Source: three-view drawing plus pictorial views. Frame: mm from the lowest corner of the part. A direction names the side the tool comes from. Round coordinates to 2 decimals unless told otherwise and drop trailing zeros. Write each loop counter-clockwise with the first axis right and the second up, starting at its lowest first coordinate (ties: lowest second). Pieces come first, ordered by that corner, then holes. Notation, with made-up numbers: M 81,43 L 123,43 A20 cw 123,69 Z; hole C 49.25,89 d4. An arc over 180 degrees is marked long. Answer as CSV lines item,"result". Start each with the question number.
Q1. Section query D-D on x = 41. Output: boundary loops of the cut face in (y, z).
Q2. Mould query, pull axis X, two halves, no side actions, for the marked faces 1 and 2. Classes: pulls with the +X half, pulls with the -X half, needs draft (parallel to the pull), parting line crosses it, or undercut.
Q3. First-contact query: pin 1 (3.5 mm diameter, centred on x = 31, y = 3.5, fed in from -Z); pin 2 (1 mm diameter, centred on y = 5, z = 5.5, fed in from -X). Flat tips, straight axial feed; report the tip coordinate or a pass-through.
Q4. Section query A-A on y = 3.5. Output: boundary loops of the cut face in (x, z).
Q5. Reachability of the marked faces 3 and 4 from +Z, -Z, +X, -X, +Y, -Y: full face, straight path, thin tool, end or side. Return the list, or none.
Q6. Section query B-B on z = 9.5. Output: boundary loops of the cut face in (x, y), and give its area (3 significant figures).
Q7. Ray query, probe 1 along Y at (x, z) = (21, 6.5); probe 2 along X at (y, z) = (2.5, 5); probe 3 along X at (y, z) = (3, 6.5). Return the intervals inside material, ascending.
Q8. Section query C-C on x = 34. Output: boundary loops of the cut face in (y, z), and give its area (3 significant figures).
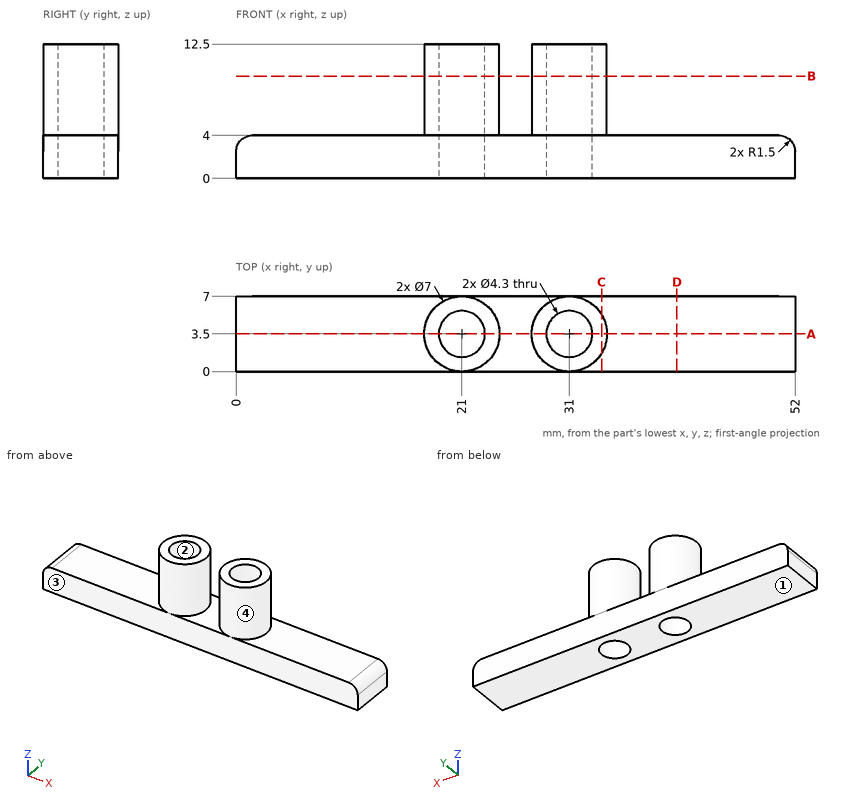
Entries:
1,outline,"M 0,0 L 7,0 L 7,4 L 0,4 Z"
2,face 1,"needs draft"
2,face 2,"undercut"
3,pin 1,"passes through"
3,pin 2,"stops at x = 17.65"
4,outline,"M 0,0 L 18.85,0 L 18.85,12.5 L 17.5,12.5 L 17.5,4 L 1.5,4 A1.5 ccw 0,2.5 Z; M 23.15,0 L 28.85,0 L 28.85,12.5 L 27.5,12.5 L 27.5,4 L 24.5,4 L 24.5,12.5 L 23.15,12.5 Z; M 33.15,0 L 52,0 L 52,2.5 A1.5 ccw 50.5,4 L 34.5,4 L 34.5,12.5 L 33.15,12.5 Z"
5,face 3,"+Z, -Z, +X, -X, -Y"
5,face 4,"+Z"
6,outline,"C 21,3.5 d7; C 31,3.5 d7; hole C 21,3.5 d4.3; hole C 31,3.5 d4.3"
6,area,"47.9 mm^2"
7,probe 1,"y = 0 to 1.35, 5.65 to 7"
7,probe 2,"x = 17.65 to 19.1, 22.9 to 24.35, 27.65 to 29.1, 32.9 to 34.35"
7,probe 3,"x = 17.54 to 18.91, 23.09 to 24.46, 27.54 to 28.91, 33.09 to 34.46"
8,outline,"M 0,0 L 7,0 L 7,4 L 5.3,4 L 5.3,12.5 L 1.7,12.5 L 1.7,4 L 0,4 Z"
8,area,"58.6 mm^2"
